Geometry check sheet. Reference: drawing and pictorial views, mm from the part's lowest x, y, z. A direction names the side the tool comes from. Give positions to 0.01 mm unless a question says otherwise; leave off trailing zeros. Order: outer loops, then holes, each group sorted by start corner. A loop starts at its lowest first (then second) coordinate and runs counter-clockwise, first axis right, second up.
Item 1: Material ranges on line 1 along Y through (x, z) = (96, 20.5); line 2 along Y through (x, z) = (80, 51); line 3 along X through (y, z) = (179, 16.5), recorded low to high.
Item 2: Gauge pin test, flat ends, axial feed: P1, Ø2, axis at x = 39.5, y = 76.5, coming from the -Z side; P2, Ø4, axis at y = 194, z = 19, coming from the -X side. Record the tip position at first contact, or that the pin passes through.
Item 3: Sectioned sample at B-B on z = 18. Record the boundary of the cut face in (x, y), and give its area (3 significant figures).
Item 4: Release check for a two-part mould opening along Y. For the marked faces 1, 2 and 3 record: released by +Y, released by -Y, zero draft, split by the parting line, or undercut.
Item 5: Sectioned sample at D-D on x = 38. Record the boundary of the cut face in (y, z), and give its area (3 significant figures).
Item 6: Sectioned sample at C-C on x = 80. Record the boundary of the cut face in (y, z).
Item 7: Access from +Z, -Z, +X, -X, +Y, -Y to the whole of each face (thin tool, end or side, straight path). Record for the marked faces 4 and 5.
Item 8: Sectioned sample at A-A on y = 125. Record the boundary of the cut face in (x, z).
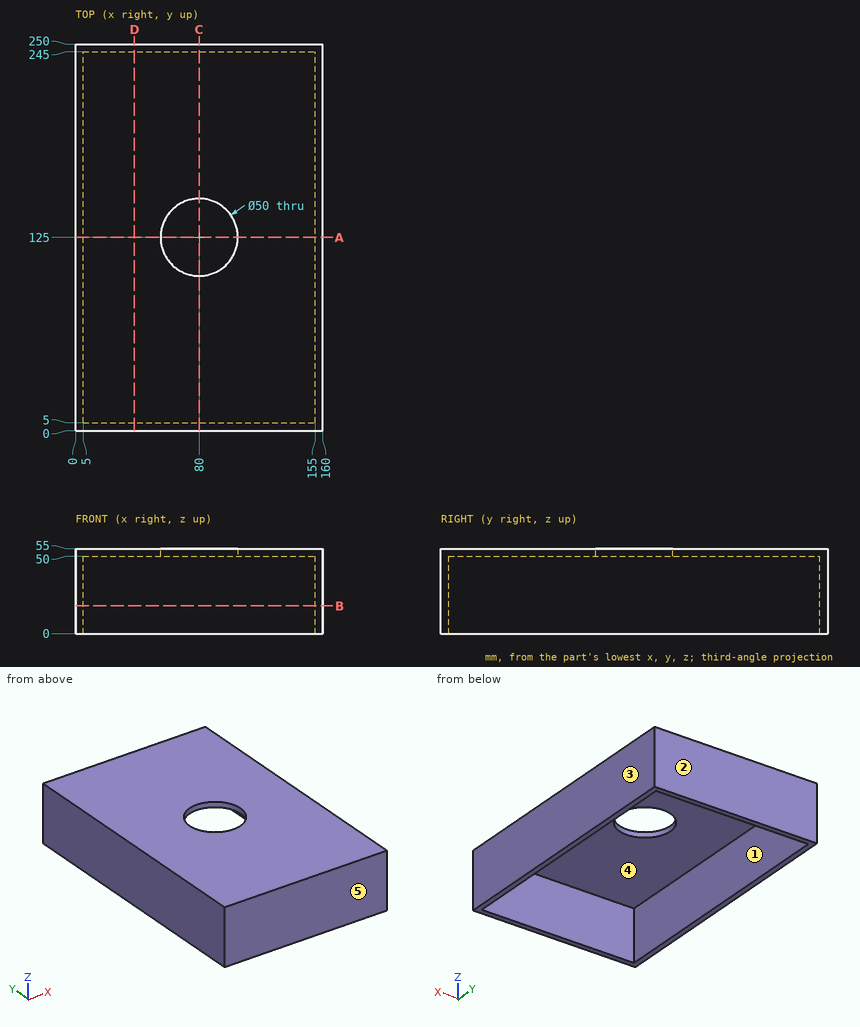
Report:
1. line 1: y = 0 to 5, 245 to 250
1. line 2: y = 0 to 100, 150 to 250
1. line 3: x = 0 to 5, 155 to 160
2. P1: stops at z = 50
2. P2: stops at x = 0
3. outline: (0, 0) - (160, 0) - (160, 250) - (0, 250) - close; hole (5, 5) - (155, 5) - (155, 245) - (5, 245) - close
3. area: 4,000 mm2
4. face 1: undercut
4. face 2: released by +Y
4. face 3: zero draft
5. outline: (0, 0) - (5, 0) - (5, 50) - (245, 50) - (245, 0) - (250, 0) - (250, 55) - (0, 55) - close
5. area: 1,750 mm2
6. outline: (0, 0) - (5, 0) - (5, 50) - (100, 50) - (100, 55) - (0, 55) - close; (150, 50) - (245, 50) - (245, 0) - (250, 0) - (250, 55) - (150, 55) - close
7. face 4: -Z
7. face 5: +Z, -Z, +X, -X, -Y
8. outline: (0, 0) - (5, 0) - (5, 50) - (55, 50) - (55, 55) - (0, 55) - close; (105, 50) - (155, 50) - (155, 0) - (160, 0) - (160, 55) - (105, 55) - close
